```python
from build123d import *

# Parameters (mm, degrees)
SKETCH_1_W      = 92
SKETCH_1_H      = 100
EXTRUDE_1_DEPTH = 34
SKETCH_2_W      = 79
SKETCH_2_H      = 39
EXTRUDE_2_DEPTH = 25
EXTRUDE_3_DEPTH = 2


with BuildPart() as part:
    # Эскиз1 → Бобышка-Вытянуть1 (new body)
    with BuildSketch(Plane(origin=(0, 0, 0), x_dir=(1, 0, 0), z_dir=(0, 1, 0))):
        with Locations((46, 50)):
            Rectangle(SKETCH_1_W, SKETCH_1_H)
    extrude(amount=EXTRUDE_1_DEPTH)

    # Эскиз2 → Бобышка-Вытянуть2 (add)
    with BuildSketch(Plane(origin=(0, 34, 0), x_dir=(1, 0, 0), z_dir=(0, 1, 0))):
        with Locations((46, 50)):
            Rectangle(SKETCH_2_W, SKETCH_2_H)
    extrude(amount=EXTRUDE_2_DEPTH)

    # Эскиз3 → Бобышка-Вытянуть3 (add)
    with BuildSketch(Plane.XZ):
        Polygon((0, 12), (18, 12), (18, 2), (24.5, 2), (24.5, 12), (42.75, 12), (42.75, 2), (49.25, 2), (49.25, 12), (67.5, 12), (67.5, 2), (74, 2), (74, 12), (92, 12), (92, -112), (74, -112), (74, -102), (67.5, -102), (67.5, -112), (49.25, -112), (49.25, -102), (42.75, -102), (42.75, -112), (24.5, -112), (24.5, -102), (18, -102), (18, -112), (0, -112), align=None)
    extrude(amount=-EXTRUDE_3_DEPTH)


solid = part.part
```
Work out the finished part from the listing and answer in its coordinate system (mm). A direction names the side the tool comes from. Give positions to 0.01 mm unless a question says otherwise; leave off trailing zeros. Loops run counter-clockwise (first coordinate to the right, second up) from the corner with the lowest first, then second, coordinate; pieces in that order, holes last. Notation, with made-up numbers: (3.5, -20) -> (62.5, -20) arc R14 ccw to (62.5, -4) -> close; hole circle Ø5 at (-27.75, 29). An arc over 180 degrees is marked (long way). Put each result on its own line as item: value. Start each with the question number.
Item 1: The part is cut by section A-A (x = 72). Give the vertices of the cut face in (y, z).
Item 2: Which of the six approach directions +Z, -Z, +X, -X, +Y, -Y give full straight-line access (tool end or side, diameter ignored) to faces 1 (the face through (6.5, 46, -50)), 2 (the face through (92, 17, -49)), 3 (the face through (47, 2, 1)), 4 (the face through (85.5, 46, -50)), 5 (the face through (45, 18, -100))?
Item 3: The part is cut by section B-B (z = -40.5). Give the vertices of the cut face in (x, y).
Item 4: Find the intervals of material crossed by L1, parallel to Z at x = 76, y = 30.5; L2, parallel to Z at x = 84, y = 49.5; L3, parallel to Y at x = 68.5, z = -86.5, in increasing order. Write a range as [from, to].
Item 5: The part is cut by section C-C (x = 30). Give the vertices of the cut face in (y, z).
Item 6: The part is cut by section D-D (y = 15.5). Give the vertices of the cut face in (x, z), then the cut area to 3 significant figures.
Item 7: Each of these flat-tipped pins is pushed along its axis until it touches: P1, Ø9.5, axis at x = 67, y = 19, coming from the -Z side; P2, Ø3, axis at x = 77, y = 15, coming from the +Z side; P3, Ø1.6, axis at x = 71, y = 0.5, coming from the +Z side. Where does it stop, or does it pass through?
Answers below:
1. outline: (0, -102) -> (2, -102) -> (2, -100) -> (34, -100) -> (34, -69.5) -> (59, -69.5) -> (59, -30.5) -> (34, -30.5) -> (34, 0) -> (2, 0) -> (2, 2) -> (0, 2) -> close
2. face 1: +Z, -Z, -X, +Y
2. face 2: +Z, -Z, +X, +Y, -Y
2. face 3: +Z, +X, -X, +Y
2. face 4: +Z, -Z, +X, +Y
2. face 5: -Z, +X, -X, +Y
3. outline: (0, 0) -> (92, 0) -> (92, 34) -> (85.5, 34) -> (85.5, 59) -> (6.5, 59) -> (6.5, 34) -> (0, 34) -> close
4. L1: [-100, 0]
4. L2: [-69.5, -30.5]
4. L3: [0, 34]
5. outline: (0, -112) -> (2, -112) -> (2, -100) -> (34, -100) -> (34, -69.5) -> (59, -69.5) -> (59, -30.5) -> (34, -30.5) -> (34, 0) -> (2, 0) -> (2, 12) -> (0, 12) -> close
6. outline: (0, -100) -> (92, -100) -> (92, 0) -> (0, 0) -> close
6. area: 9,200 mm2
7. P1: z = -100
7. P2: z = 0
7. P3: z = 2
